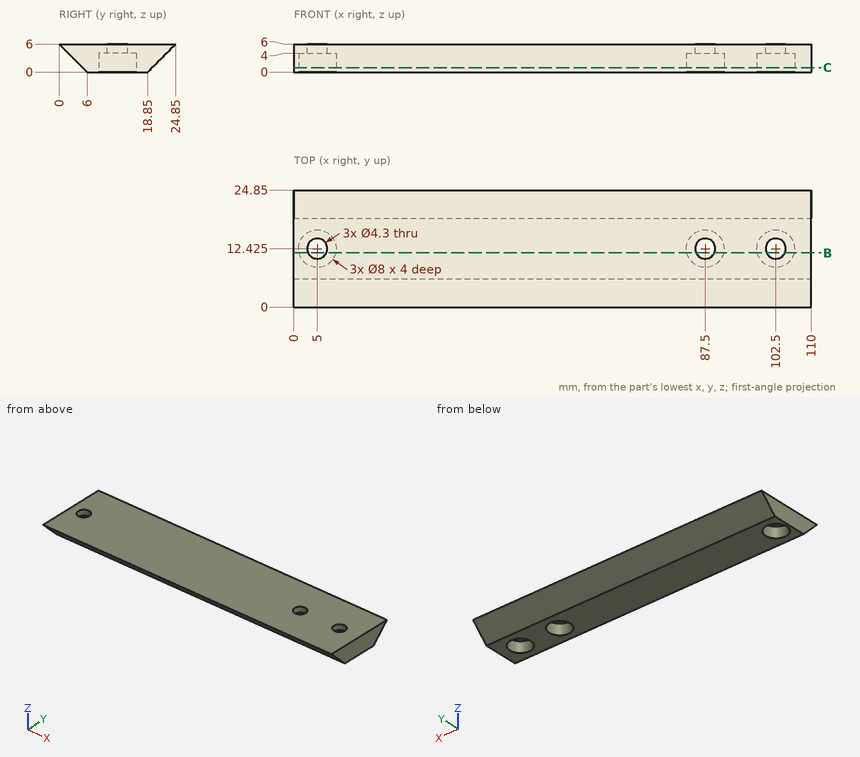
Answer from the drawing. Dimensions are ordinates in mm from the lowest x, y and z of the part. Coordinates: 2 decimals unless noted, no trailing zeros. Order: outer loops, then holes, each group sorted by start corner. A loop starts at its lowest first (then second) coordinate and runs counter-clockwise, first axis right, second up. Notation, with made-up numbers: M 52,-8.75 L 70,-8.75 A32 ccw 70,26.25 Z; hole C 15.25,-24.75 d11. An arc over 180 degrees is marked long. Put each result on its own line as item: value. Start each with the question number.
Item 1: Consider probe 1 along X at (y, z) = (10, 3.25); probe 2 along Z at (x, y) = (9.5, 2); probe 3 along X at (y, z) = (9.75, 2). Determine where each line is inside the solid, lowest interval first. Write a range as [from, to].
Item 2: Section C-C, the plane z = 1 is taken. Determine the outline of the cut face in (x, y) (3 decimals).
Item 3: Section B-B, the plane y = 11.5 is taken. Determine the outline of the cut face in (x, z).
Item 4: Given pin 1 Ø1 at (x, z) = (31.5, 4.5) entering from -Y; pin 2 Ø4 at (x, y) = (103, 13) entering from -Z, each flat-ended and moving along its own axis, determine where each tip first touches the part or whether it passes through.
Computed:
1. probe 1: x = [0, 1.82], [8.18, 84.32], [90.68, 99.32], [105.68, 110]
1. probe 2: z = [4, 6]
1. probe 3: x = [0, 2.03], [7.97, 84.53], [90.47, 99.53], [105.47, 110]
2. outline: M 0,5 L 110,5 L 110,19.85 L 0,19.85 Z; hole C 5,12.425 d8; hole C 87.5,12.425 d8; hole C 102.5,12.425 d8
3. outline: M 0,0 L 1.11,0 L 1.11,4 L 3.06,4 L 3.06,6 L 0,6 Z; M 6.94,4 L 8.89,4 L 8.89,0 L 83.61,0 L 83.61,4 L 85.56,4 L 85.56,6 L 6.94,6 Z; M 89.44,4 L 91.39,4 L 91.39,0 L 98.61,0 L 98.61,4 L 100.56,4 L 100.56,6 L 89.44,6 Z; M 104.44,4 L 106.39,4 L 106.39,0 L 110,0 L 110,6 L 104.44,6 Z
4. pin 1: stops at y = 1
4. pin 2: stops at z = 4
